from build123d import *

# Parameters (mm, degrees)
F0_W           = 29.3
F0_H           = 11.3
F2_W           = 24.5
F2_H           = 11
F6_D           = 4
F6_CBORE_D     = 7
F6_CBORE_DEPTH = 3
F7_R           = 4
F8_DEPTH       = 5.6510001
F8_DEPTH_BACK  = 4


with BuildPart() as f3:
    # F0 (on Top) → F3 section 0
    with BuildSketch(Plane.XY):
        Rectangle(F0_W, F0_H)
    # F2 (on offset) → F3 section 1
    with BuildSketch(Plane.XY.offset(14)):
        Rectangle(F2_W, F2_H)
    loft()

    # F6 (through all)
    with Locations(Plane.XY.offset(14)):
        with Locations((-8.15, 0), (8.15, 0)):
            CounterBoreHole(F6_D / 2, F6_CBORE_D / 2, F6_CBORE_DEPTH)

    # F7 (on Front) → F8 (cut, two sides)
    with BuildSketch(Plane.XZ) as f8_sk:
        with Locations((0, 7.9)):
            Circle(F7_R)
    extrude(amount=F8_DEPTH, mode=Mode.SUBTRACT)
    extrude(f8_sk.sketch, amount=-F8_DEPTH_BACK, mode=Mode.SUBTRACT)


solid = f3.part
The listing builds one solid part. Answer for the finished solid, in the listing's coordinates (mm). A direction names the side the tool comes from. Give positions to 0.01 mm unless a question says otherwise; leave off trailing zeros. Use a Markdown table: item, result.
1. A tool of negligible diameter and unlimited length cuts with its end or side. For faces 4 (the cylindrical face through (-0.867, -0.737, 3.995)), 5 (the flat face through (0, 0, 0)), 6 (the flat face through (10, -2, 11)), from which of +Z, -Z, +X, -X, +Y, -Y can it reach the whole face along a straight path? Write none if from no direction.
Values follow:
| item | result |
|---|---|
| face 4 | -Y |
| face 5 | -Z, +X, -X, +Y, -Y |
| face 6 | +Z |
2. Section A-A on y = 0 is taken. Count the separate pieces of the cut face and the enclosed holes in it, plus the area to 3 significant figures.
Values follow:
| item | result |
|---|---|
| separate pieces | 3 |
| enclosed holes | 1 |
| area | 196 mm² |
3. Each of these flat-tipped pins is pushed along its axis until it touches: P1, Ø5, axis at x = -0.5, z = 8.5, coming from the +Y side; P2, Ø6.5, axis at x = -0.5, z = 6, coming from the -Y side; P3, Ø2, axis at x = 6.5, y = 0.5, coming from the +Z side. Where does it stop, or does it pass through?
Values follow:
| item | result |
|---|---|
| P1 | stops at y = 5.59 |
| P2 | stops at y = -5.62 |
| P3 | stops at z = 11 |
4. For a pull along X with two mould halves and no side action, classify faces 1 (the cylindrical face through (9.737, -1.217, 5.423)), 2 (the flat face through (0, 0, 14)), 3 (the cylindrical face through (-6.152, 0.088, 5.423)) as released by +X, released by -X, zero draft, split by the parting line, or undercut.
Values follow:
| item | result |
|---|---|
| face 1 | undercut |
| face 2 | zero draft |
| face 3 | undercut |
5. Find the intervals of material crossed by probe 1 along X at (y, z) = (-0.5, 12.75); probe 2 along X at (y, z) = (2.25, 13); probe 3 along X at (y, z) = (0.75, 7.9), in increasing order. Write a range as from..to.
Values follow:
| item | result |
|---|---|
| probe 1 | x = -12.46..-11.61, -4.69..4.69, 11.61..12.46 |
| probe 2 | x = -12.42..-10.83, -5.47..5.47, 10.83..12.42 |
| probe 3 | x = -13.3..-10, -6.3..-4, 4..6.3, 10..13.3 |
